Build history of the part. All positions in model axes, mm. A direction names the side the tool comes from. Round coordinates to 2 decimals unless told otherwise and drop trailing zeros. Write each loop counter-clockwise with the first axis right and the second up, starting at its lowest first coordinate (ties: lowest second). Pieces come first, ordered by that corner, then holes.
Item 1: Band-saw the part on A-A, the plane z = -98. Write the cut outline in (x, y), then the cut area to 3 significant figures.
Item 2: Band-saw the part on B-B, the plane y = 65. Write the cut outline in (x, z).
Item 3: Drop flat-ended pins along their axis: pin 1 Ø5 at (y, z) = (57.5, -43.5) entering from -X; pin 2 Ø3 at (y, z) = (-81, -98.5) entering from -X; pin 3 Ø10 at (x, z) = (9.5, 12) entering from -Y. Give the stop position or say it passes through.
Item 4: Wall check: probe 1 along X at (y, z) = (0, 80.5); probe 2 along Z at (x, y) = (-79, -14); probe 3 along Y at (x, z) = (19, -61.5). Give the ranges that are in metal, low to high.
Item 5: Mould opens along Z. For faces 4 (the flat face through (-25, -74, 155)), 5 (the flat face through (47, -25, 150)), 6 (the cylindrical face through (-31.54, -100.15, -169.72)) say: +Z half, -Z half, draft (parallel to the pull), parting line (faces both ways), or undercut.
Item 6: 3-axis set-ups, long thin cutter, end or side, ignore diameter. For faces 1 (the flat face through (-18.8, -73.3, 160)), 2 (the flat face through (77, 24, -150)), 3 (the cylindrical face through (50.44, 65.79, 157.54)): which of +Z, -Z, +X, -X, +Y, -Y reach the whole face in a straight line?
```python
from build123d import *

# Parameters (mm, degrees)
SKETCH4_R          = 25
CUT_EXTRUDE1_DEPTH = 350
CHAMFER1_SIZE      = 4


with BuildPart() as part:
    # Sketch2 → Revolve1 (revolve)
    with BuildSketch(Plane(origin=(0, 0, 0), x_dir=(0, 0, -1), z_dir=(1, 0, 0)), mode=Mode.PRIVATE) as revolve1_sk:
        Polygon((190, 0), (190, 105), (150, 105), (150, 79.9), (120, 79.9), (120, 87.9), (-125, 87.9), (-125, 77.9), (-155, 77.9), (-155, 82.9), (-160, 82.9), (-160, 75.5), (150, 75.5), (150, 57.5), (-150, 57.5), (-150, 52.5), (-160, 52.5), (-160, 0), align=None)
    revolve(revolve1_sk.sketch.rotate(Axis((0, 0, 160), (0, 0, -1)), 180), axis=Axis((0, 0, 160), (0, 0, -1)))

    # Sketch4 → Cut-Extrude1 (cut)
    with BuildSketch(Plane(origin=(0, 0, -190), x_dir=(-1, 0, 0), z_dir=(0, 0, -1))):
        with Locations(Location((0, 0, 0), (0, 0, 90))):
            Circle(SKETCH4_R)
    extrude(amount=-CUT_EXTRUDE1_DEPTH, mode=Mode.SUBTRACT)

    # Chamfer1
    chamfer1_edges = [part.edges().sort_by_distance(p)[0] for p in [
        (0, -25, 160),
    ]]
    chamfer(chamfer1_edges, length=CHAMFER1_SIZE)


solid = part.part
```
Results:
1. outline: circle Ø175.8 at (0, 0); circle Ø115 at (0, 0); hole circle Ø151 at (0, 0); hole circle Ø50 at (0, 0)
1. area: 14,800 mm2
2. outline: (-82.46, -190) - (82.46, -190) - (82.46, -150) - (46.47, -150) - (46.47, -120) - (59.17, -120) - (59.17, 125) - (42.93, 125) - (42.93, 155) - (51.45, 155) - (51.45, 160) - (38.41, 160) - (38.41, -150) - (-38.41, -150) - (-38.41, 160) - (-51.45, 160) - (-51.45, 155) - (-42.93, 155) - (-42.93, 125) - (-59.17, 125) - (-59.17, -120) - (-46.47, -120) - (-46.47, -150) - (-82.46, -150) - close
3. pin 1: stops at x = -68.57
3. pin 2: stops at x = -37.5
3. pin 3: stops at y = -87.78
4. probe 1: x = -87.9 to -75.5, -57.5 to -25, 25 to 57.5, 75.5 to 87.9
4. probe 2: z = -190 to -150, -120 to 125, 155 to 160
4. probe 3: y = -85.82 to -73.07, -54.27 to -16.25, 16.25 to 54.27, 73.07 to 85.82
5. face 4: undercut
5. face 5: +Z half
5. face 6: draft
6. face 1: +Z, +X, -X, +Y, -Y
6. face 2: none
6. face 3: +Z
